Verification items for this drawing (mm, ordinates from the low corner). A direction names the side the tool comes from. Give positions to 0.01 mm unless a question says otherwise; leave off trailing zeros. Loops run counter-clockwise (first coordinate to the right, second up) from the corner with the lowest first, then second, coordinate; pieces in that order, holes last. Notation, with made-up numbers: (44.25, -29.75) -> (59.25, -29.75) arc R12 ccw to (59.25, -7.75) -> close; hole circle Ø11 at (45, 9). An arc over 180 degrees is marked (long way). Write each question's results on one line, items separated by ' | '. Start each with the question number.
1) Depth check by flat-ended pin: pin 1 (2 mm diameter, centred on x = 13.5, y = 50.5, fed in from -Z); pin 2 (3.5 mm diameter, centred on x = 12, z = 6, fed in from +Y); pin 3 (1.8 mm diameter, centred on x = 10, y = 20, fed in from -Z); pin 4 (2.5 mm diameter, centred on x = 10, z = 32, fed in from -Y). Enter the tip coordinate at first touch or a pass-through.
2) Sectioned sample at D-D on x = 2.75. Record the cut outline in (y, z), then the cut area to 3 significant figures.
3) Sectioned sample at A-A on z = 10. Record the cut outline in (x, y), then the cut area to 3 significant figures.
4) Set-up check for the marked faces 4, 5 and 6: record each of +Z, -Z, +X, -X, +Y, -Y from which the full face is reachable in a straight line by a thin tool's end or side.
5) Scan lines: line 1 (Z direction, x = 15, y = 36.5); line 2 (Y direction, x = 7.75, z = 32.5); line 3 (X direction, y = 1.35, z = 10). Record each from-to range of solid material in increasing order. Write a range as from..to.
6) Sectioned sample at C-C on x = 10. Count the separate pieces of the cut face and the enclosed holes in it, then the cut area to 3 significant figures.
7) Sectioned sample at B-B on y = 38. Record the cut outline in (x, z).
8) Draft check along Y on the marked faces 1, 2 and 3. Enter one of: pulls with the +Y half, pulls with the -Y half, needs draft (parallel to the pull), parting line crosses it, or undercut.
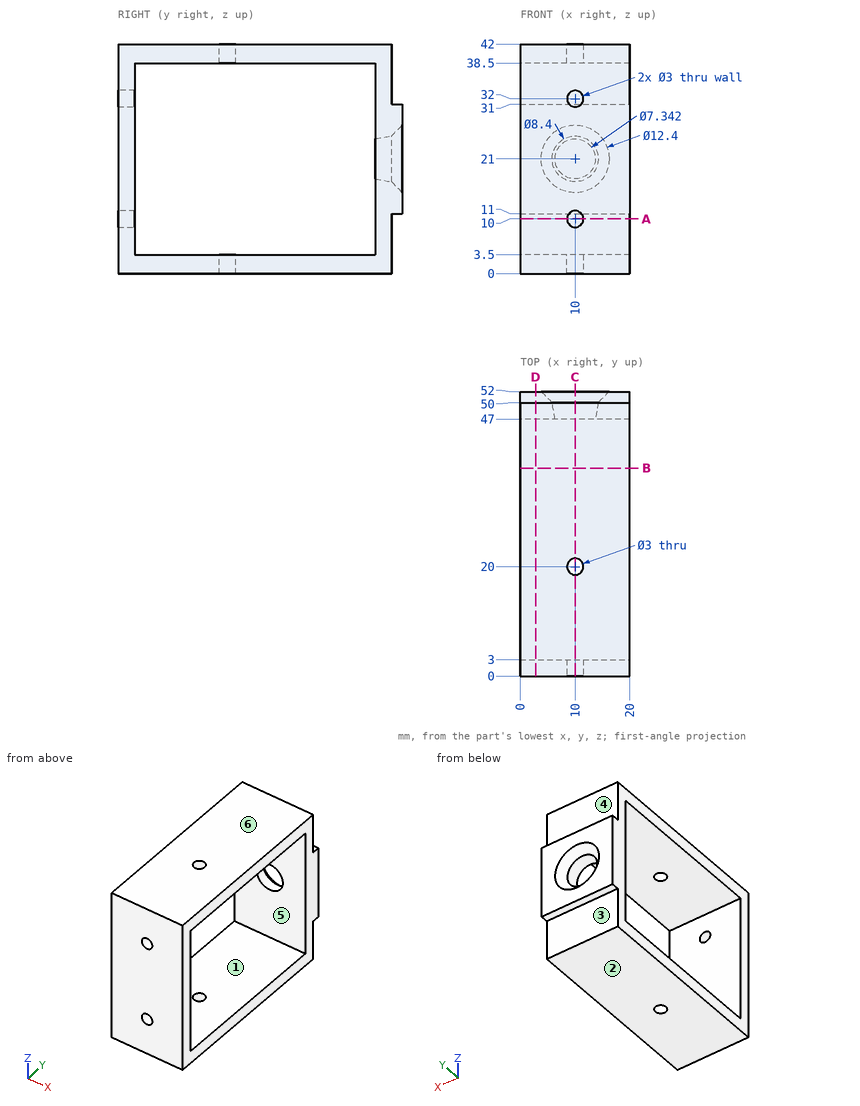
Result:
1) pin 1: z = 0 | pin 2: y = 50 | pin 3: through | pin 4: y = 47
2) outline: (0, 0) -> (50, 0) -> (50, 11) -> (52, 11) -> (52, 31) -> (50, 31) -> (50, 42) -> (0, 42) -> close; hole (3, 3.5) -> (47, 3.5) -> (47, 38.5) -> (3, 38.5) -> close | area: 600 mm^2
3) outline: (0, 0) -> (8.5, 0) -> (8.5, 3) -> (0, 3) -> close; (0, 47) -> (20, 47) -> (20, 50) -> (0, 50) -> close; (11.5, 0) -> (20, 0) -> (20, 3) -> (11.5, 3) -> close | area: 111 mm^2
4) face 4: +Z, +X, -X, +Y | face 5: +X, -X | face 6: +Z, +X, -X, +Y, -Y
5) line 1: 0..3.5, 38.5..42 | line 2: 0..3, 47..50 | line 3: 0..8.5, 11.5..20
6) separate pieces: 5 | enclosed holes: 0 | area: 517 mm^2
7) outline: (0, 0) -> (20, 0) -> (20, 3.5) -> (0, 3.5) -> close; (0, 38.5) -> (20, 38.5) -> (20, 42) -> (0, 42) -> close
8) face 1: undercut | face 2: needs draft | face 3: pulls with the +Y half
